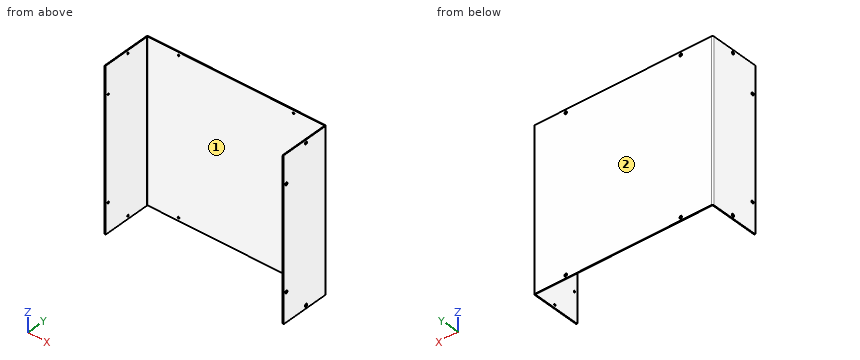
```python
from build123d import *

# Parameters (mm, degrees)
FLANGE_BASE1_DEPTH                   = 390
ESBO_O6_R                            = 2
CORTE_EXTRUS_O1_DEPTH                = 558
ESBO_O7_R                            = 2
CORTE_EXTRUS_O2_DEPTH                = 558
QUEBRA_CANTO1_START                  = -2
QUEBRA_CANTO1_DEPTH                  = 435.6
ESCAREADO_PARA_SFHCS_M41_D           = 4
ESCAREADO_PARA_SFHCS_M41_CSINK_D     = 6.5
ESCAREADO_PARA_SFHCS_M41_CSINK_ANGLE = 90
ESCAREADO_PARA_SFHCS_M42_D           = 4
ESCAREADO_PARA_SFHCS_M42_CSINK_D     = 6.5
ESCAREADO_PARA_SFHCS_M42_CSINK_ANGLE = 90
ESCAREADO_PARA_SFHCS_M43_D           = 4
ESCAREADO_PARA_SFHCS_M43_CSINK_D     = 6.5
ESCAREADO_PARA_SFHCS_M43_CSINK_ANGLE = 90


# Read off the part's stored shape, not the designer's step: Quebra-Canto1
# Sheet-metal steps are written as plain solids
with BuildPart() as part:
    # Esboço1 → Flange-base1 (new body)
    with BuildSketch(Plane.XY):
        with BuildLine():
            Line((0, 0), (0, 119.8))
            ThreePointArc((0, 119.8), (0.351471863, 120.648528137), (1.2, 121))
            Line((1.2, 121), (430.4, 121))
            ThreePointArc((430.4, 121), (431.248528137, 120.648528137), (431.6, 119.8))
            Line((431.6, 119.8), (431.6, 0))
            Line((431.6, 0), (433.6, 0))
            Line((433.6, 0), (433.6, 119.8))
            ThreePointArc((433.6, 119.8), (432.6627417, 122.0627417), (430.4, 123))
            Line((430.4, 123), (1.2, 123))
            ThreePointArc((1.2, 123), (-1.0627417, 122.0627417), (-2, 119.8))
            Line((-2, 119.8), (-2, 0))
            Line((-2, 0), (0, 0))
        make_face()
    extrude(amount=FLANGE_BASE1_DEPTH)

    # Esboço6 → Corte-extrusão1 (cut)
    with BuildSketch(Plane(origin=(433.6, 0, 0), x_dir=(0, 0, -1), z_dir=(1, 0, 0))):
        with Locations(Location((-382.5, 65, 0), (0, 0, 180))):
            Circle(ESBO_O6_R)
        with Locations(Location((-320, 8.4, 0), (0, 0, 180))):
            Circle(ESBO_O6_R)
        with Locations(Location((-70, 8.4, 0), (0, 0, 180))):
            Circle(ESBO_O6_R)
        with Locations(Location((-7.5, 65, 0), (0, 0, 180))):
            Circle(ESBO_O6_R)
    extrude(amount=-CORTE_EXTRUS_O1_DEPTH, mode=Mode.SUBTRACT)

    # Esboço7 → Corte-extrusão2 (cut)
    with BuildSketch(Plane(origin=(0, 123, 0), x_dir=(1, 0, 0), z_dir=(0, 1, 0))):
        with Locations(Location((75.8, -7.5, 0), (0, 0, 270))):
            Circle(ESBO_O7_R)
        with Locations(Location((355.8, -7.5, 0), (0, 0, 270))):
            Circle(ESBO_O7_R)
        with Locations(Location((355.8, -382.5, 0), (0, 0, 270))):
            Circle(ESBO_O7_R)
        with Locations(Location((75.8, -382.5, 0), (0, 0, 270))):
            Circle(ESBO_O7_R)
    extrude(amount=-CORTE_EXTRUS_O2_DEPTH, mode=Mode.SUBTRACT)

    # Quebra-Canto1 outline → Quebra-Canto1 (cut)
    with BuildSketch(Plane.YZ.offset(QUEBRA_CANTO1_START)):
        with BuildLine():
            Line((0, 390), (0, 388))
            ThreePointArc((0, 388), (0.585786438, 389.414213562), (2, 390))
            Line((2, 390), (0, 390))
        make_face()
        with BuildLine():
            ThreePointArc((2, 0), (0.585786438, 0.585786438), (0, 2))
            Line((0, 2), (0, 0))
            Line((0, 0), (2, 0))
        make_face()
    extrude(amount=QUEBRA_CANTO1_DEPTH, mode=Mode.SUBTRACT)

    # Escareado para SFHCS M41 (through all)
    with Locations(Plane(origin=(0, 123, 0), x_dir=(1, 0, 0), z_dir=(0, 1, 0))):
        with Locations((75.8, -382.5), (355.8, -382.5), (355.8, -7.5), (75.8, -7.5)):
            CounterSinkHole(ESCAREADO_PARA_SFHCS_M41_D / 2, ESCAREADO_PARA_SFHCS_M41_CSINK_D / 2, counter_sink_angle=ESCAREADO_PARA_SFHCS_M41_CSINK_ANGLE)

    # Escareado para SFHCS M42 (through all)
    with Locations(Plane.ZY.offset(2)):
        with Locations((382.5, 65), (320, 8.4), (7.5, 65), (70, 8.4)):
            CounterSinkHole(ESCAREADO_PARA_SFHCS_M42_D / 2, ESCAREADO_PARA_SFHCS_M42_CSINK_D / 2, counter_sink_angle=ESCAREADO_PARA_SFHCS_M42_CSINK_ANGLE)

    # Escareado para SFHCS M43 (through all)
    with Locations(Plane(origin=(433.6, 65, 382.5), x_dir=(0, 1, 0), z_dir=(1, 0, 0))):
        with Locations((0, 0), (-56.6, -62.5), (-56.6, -312.5), (0, -375)):
            CounterSinkHole(ESCAREADO_PARA_SFHCS_M43_D / 2, ESCAREADO_PARA_SFHCS_M43_CSINK_D / 2, counter_sink_angle=ESCAREADO_PARA_SFHCS_M43_CSINK_ANGLE)


solid = part.part
```
Build history of the part. All positions in model axes, mm. Face numbers are marked on the shaded views. A direction names the side the tool comes from. Coordinates: 2 decimals unless noted, no trailing zeros. Write each loop counter-clockwise with the first axis right and the second up, starting at its lowest first coordinate (ties: lowest second). Pieces come first, ordered by that corner, then holes.
1. 3-axis set-ups, long thin cutter, end or side, ignore diameter. For the marked faces 1 and 2: which of +Z, -Z, +X, -X, +Y, -Y reach the whole face in a straight line?
Answer block:
face 1: +Z, -Z, -Y
face 2: +Z, -Z, +X, -X, +Y
2. Band-saw the part on C-C, the plane x = 407. Give the cut face in (y, z), and give its area (3 significant figures).
Answer block:
outline: (121, 0) - (123, 0) - (123, 390) - (121, 390) - close
area: 780 mm2
3. Drop flat-ended pins along their axis: pin 1 (4.5 mm diameter, centred on y = 8.4, z = 320, fed in from +X); pin 2 (1 mm diameter, centred on x = 213.5, z = 326, fed in from -Y); pin 3 (5 mm diameter, centred on y = 65, z = 7.5, fed in from +X). Give the stop position or say it passes through.
Answer block:
pin 1: stops at x = 432.6
pin 2: stops at y = 121
pin 3: stops at x = 432.85
4. Band-saw the part on B-B, the plane z = 185. Give the cut face in (x, y).
Answer block:
outline: (-2, 0) - (0, 0) - (0, 119.8) arc R1.2 cw to (1.2, 121) - (430.4, 121) arc R1.2 cw to (431.6, 119.8) - (431.6, 0) - (433.6, 0) - (433.6, 119.8) arc R3.2 ccw to (430.4, 123) - (1.2, 123) arc R3.2 ccw to (-2, 119.8) - close
5. Drill centre lines: probe 1 along Z at (x, y) = (355.8, 121.35); probe 2 along Z at (x, y) = (432.1, 8.4); probe 3 along X at (y, z) = (116, 128). Where is each one in solid material? Low to high.
Answer block:
probe 1: z = 0 to 5.5, 9.5 to 380.5, 384.5 to 390
probe 2: z = 0 to 68, 72 to 318, 322 to 390
probe 3: x = -2 to 0, 431.6 to 433.6
6. Band-saw the part on A-A, the plane y = 98. Give the cut face in (x, z), and give its area (3 significant figures).
Answer block:
outline: (-2, 0) - (0, 0) - (0, 390) - (-2, 390) - close; (431.6, 0) - (433.6, 0) - (433.6, 390) - (431.6, 390) - close
area: 1,560 mm2
